Autodesk Inventor part; units mm, degrees
ref_plane "Work Plane7" through (3.7071, 39.9, 0.5) normal (0, 1, 0) x (1, 0, 0)
ref_plane "YZ Plane" through (0, 0, 0) normal (1, 0, 0) x (0, 1, 0)
ref_plane "XZ Plane" through (0, 0, 0) normal (0, 1, 0) x (-1, 0, 0)
ref_plane "Work Plane7" through (3.7071, 39.9, 0.5) normal (0, 1, 0) x (1, 0, 0)
sketch "Sketch4" plane through (3.7071, 39.9, 0.5) normal (0, 1, 0) x (1, 0, 0)
  circle A0 centre (6.2928, -9.3) radius 2.9
  circle A1 centre (6.2928, -9.3) radius 2.65
  line L0 (6.2928, -9.3) -> (6.2928, -8.1563)
  circle A2 centre (6.2928, -9.3) radius 1.5
  line L1 (5.9607, -6.6709) -> (6.3303, -6.4003)
  line L2 (6.6249, -6.6709) -> (6.3303, -6.4003)
  line L3 (5.3173, -6.8361) -> (5.608, -6.482)
  line L4 (5.9607, -6.6709) -> (5.608, -6.482)
  line L5 (4.7352, -7.1561) -> (4.9287, -6.7409)
  line L6 (5.3173, -6.8361) -> (4.9287, -6.7409)
  line L7 (4.2509, -7.6109) -> (4.3351, -7.1605)
  line L8 (4.7352, -7.1561) -> (4.3351, -7.1605)
  line L9 (3.895, -8.1717) -> (3.8646, -7.7146)
  line L10 (4.2509, -7.6109) -> (3.8646, -7.7146)
  line L11 (3.6897, -8.8035) -> (3.5466, -8.3682)
  line L12 (3.895, -8.1717) -> (3.5466, -8.3682)
  line L13 (3.648, -9.4664) -> (3.4011, -9.0805)
  line L14 (3.6897, -8.8035) -> (3.4011, -9.0805)
  line L15 (3.7725, -10.1189) -> (3.4374, -9.8065)
  line L16 (3.648, -9.4664) -> (3.4374, -9.8065)
  line L17 (4.0553, -10.72) -> (3.653, -10.5007)
  line L18 (3.7725, -10.1189) -> (3.653, -10.5007)
  line L19 (4.4787, -11.2318) -> (4.0346, -11.1195)
  line L20 (4.0553, -10.72) -> (4.0346, -11.1195)
  line L21 (5.0161, -11.6222) -> (4.558, -11.6239)
  line L22 (4.4787, -11.2318) -> (4.558, -11.6239)
  line L23 (5.6338, -11.8668) -> (5.1904, -11.9823)
  line L24 (5.0161, -11.6222) -> (5.1904, -11.9823)
  line L25 (6.2928, -11.95) -> (5.8921, -12.1722)
  line L26 (5.6338, -11.8668) -> (5.8921, -12.1722)
  line L27 (6.9518, -11.8668) -> (6.619, -12.1816)
  line L28 (6.2928, -11.95) -> (6.619, -12.1816)
  line L29 (7.5694, -11.6222) -> (7.3254, -12.01)
  line L30 (6.9518, -11.8668) -> (7.3254, -12.01)
  line L31 (8.1068, -11.2318) -> (7.9668, -11.6681)
  line L32 (7.5694, -11.6222) -> (7.9668, -11.6681)
  line L33 (8.5303, -10.72) -> (8.5032, -11.1773)
  line L34 (8.1068, -11.2318) -> (8.5032, -11.1773)
  line L35 (8.8131, -10.1189) -> (8.9006, -10.5687)
  line L36 (8.5303, -10.72) -> (8.9006, -10.5687)
  line L37 (8.9376, -9.4664) -> (9.1341, -9.8803)
  line L38 (8.8131, -10.1189) -> (9.1341, -9.8803)
  line L39 (8.8959, -8.8035) -> (9.1892, -9.1554)
  line L40 (8.9376, -9.4664) -> (9.1892, -9.1554)
  line L41 (8.6906, -8.1717) -> (9.0622, -8.4397)
  line L42 (8.8959, -8.8035) -> (9.0622, -8.4397)
  line L43 (8.3346, -7.6109) -> (8.7613, -7.778)
  line L44 (8.6906, -8.1717) -> (8.7613, -7.778)
  line L45 (7.8504, -7.1561) -> (8.3052, -7.2119)
  line L46 (8.3346, -7.6109) -> (8.3052, -7.2119)
  line L47 (7.2683, -6.8361) -> (7.7227, -6.777)
  line L48 (7.8504, -7.1561) -> (7.7227, -6.777)
  line L49 (6.6249, -6.6709) -> (7.0503, -6.5007)
  line L50 (7.2683, -6.8361) -> (7.0503, -6.5007)
  line L51 (-48.7072, 67.5) -> (-9.1072, 67.5)
  line L52 (-9.1072, 67.5) -> (-9.1072, 47.9)
  line L53 (-9.1072, 47.9) -> (-48.7072, 47.9)
  line L54 (-48.7072, 47.9) -> (-48.7072, 67.5)
  line L55 (-9.6072, 67.8) -> (-48.2072, 67.8)
  line L56 (-49.0072, 67) -> (-49.0072, 48.4)
  line L57 (-48.2072, 47.6) -> (-9.6072, 47.6)
  line L58 (-8.8072, 48.4) -> (-8.8072, 67)
  arc A3 (-48.2072, 67.8) -> (-49.0072, 67) centre (-48.2072, 67) ccw
  arc A4 (-49.0072, 48.4) -> (-48.2072, 47.6) centre (-48.2072, 48.4) ccw
  arc A5 (-8.8072, 67) -> (-9.6072, 67.8) centre (-9.6072, 67) ccw
  arc A6 (-9.6072, 47.6) -> (-8.8072, 48.4) centre (-9.6072, 48.4) ccw
  circle A7 centre (-38.7072, 57.7) radius 2.8043
  line L59 (-28.9072, 67.5) -> (-28.9072, 60.5718)
  arc A8 (-51.4012, 75.2248) -> (-53.5593, 41.3351) centre (-51.641, 58.2265) ccw
  arc A9 (14.1928, -9.3) -> (-1.6072, -9.3) centre (6.2928, -9.3) ccw
  line L60 (-53.5593, 41.3351) -> (-46.7288, 40.1839) construction
  line L61 (-46.7288, 40.1839) -> (-26.4146, 41.3143) construction
  line L62 (-26.4146, 41.3143) -> (-16.8338, 33.5272) construction
  line L63 (-16.8338, 33.5272) -> (-7.2254, 12.1154) construction
  line L64 (-7.2254, 12.1154) -> (-2.9491, -1.4) construction
  line L65 (-2.9491, -1.4) -> (-1.6072, -5.4747) construction
  line L66 (-1.6072, -5.4747) -> (-1.6072, -9.3) construction
  spline S0 degree 4 poles (-53.5593, 41.3351) (-46.7288, 40.1839) (-26.4146, 41.3143) (-16.8338, 33.5272) (-7.2254, 12.1154) (-2.9491, -1.4) (-1.6072, -5.4747) (-1.6072, -9.3) knots 1 1 1 1 1 2 3 4 5 5 5 5 5
  line L67 (61.2928, 67.5) -> (21.6928, 67.5)
  line L68 (21.6928, 67.5) -> (21.6928, 47.9)
  line L69 (21.6928, 47.9) -> (61.2928, 47.9)
  line L70 (61.2928, 47.9) -> (61.2928, 67.5)
  line L71 (22.1928, 67.8) -> (60.7928, 67.8)
  line L72 (61.5928, 67) -> (61.5928, 48.4)
  line L73 (60.7928, 47.6) -> (22.1928, 47.6)
  line L74 (21.3928, 48.4) -> (21.3928, 67)
  arc A10 (61.5928, 67) -> (60.7928, 67.8) centre (60.7928, 67) ccw
  arc A11 (60.7928, 47.6) -> (61.5928, 48.4) centre (60.7928, 48.4) ccw
  arc A12 (22.1928, 67.8) -> (21.3928, 67) centre (22.1928, 67) ccw
  arc A13 (21.3928, 48.4) -> (22.1928, 47.6) centre (22.1928, 48.4) ccw
  circle A14 centre (51.2928, 57.7) radius 2.8043
  line L75 (41.4928, 67.5) -> (41.4928, 60.5718)
  arc A15 (66.1449, 41.3351) -> (63.9868, 75.2248) centre (64.2266, 58.2265) ccw
  line L76 (66.1449, 41.3351) -> (59.3144, 40.1839) construction
  line L77 (59.3144, 40.1839) -> (39.0002, 41.3143) construction
  line L78 (39.0002, 41.3143) -> (29.4194, 33.5272) construction
  line L79 (29.4194, 33.5272) -> (19.811, 12.1154) construction
  line L80 (19.811, 12.1154) -> (15.5347, -1.4) construction
  line L81 (15.5347, -1.4) -> (14.1928, -5.4747) construction
  line L82 (14.1928, -5.4747) -> (14.1928, -9.3) construction
  spline S1 degree 4 poles (66.1449, 41.3351) (59.3144, 40.1839) (39.0002, 41.3143) (29.4194, 33.5272) (19.811, 12.1154) (15.5347, -1.4) (14.1928, -5.4747) (14.1928, -9.3) knots 1 1 1 1 1 2 3 4 5 5 5 5 5
  arc A16 (-1.6072, -9.3) -> (14.1928, -9.3) centre (6.2928, -9.3) ccw
  circle A17 centre (-53.6572, 62.7) radius 1.5
  line L83 (-49.0072, 57.7) -> (-54.6618, 57.7)
  circle A18 centre (-53.6572, 52.7) radius 1.5
  circle A19 centre (66.2428, 62.7) radius 1.5
  circle A20 centre (66.2428, 52.7) radius 1.5
  circle A21 centre (6.2928, -9.3) radius 4.95
  line L84 (-4.1572, 57.7) -> (-3.4323, 57.7)
  circle A22 centre (-4.1572, 57.7) radius 1.5
  circle A23 centre (16.7428, 57.7) radius 1.5
  line L85 (-51.4012, 75.2248) -> (63.9868, 75.2248)
  circle A24 centre (6.2928, -9.3) radius 9.5
  line L86 (-3.2072, -9.3) -> (-3.2072, -6.2163) construction
  line L87 (-3.2072, -6.2163) -> (-3.7947, -2.1829) construction
  line L88 (-3.7947, -2.1829) -> (-5.6572, 5.3052) construction
  line L89 (-5.6572, 5.3052) -> (-8.4358, 13.8026) construction
  spline S2 degree 4 poles (-3.2072, -9.3) (-3.2072, -6.2163) (-3.7947, -2.1829) (-5.6572, 5.3052) (-8.4358, 13.8026) knots 1 1 1 1 1 2 2 2 2 2
  line L90 (15.7928, -9.3) -> (15.7928, -6.2163) construction
  line L91 (15.7928, -6.2163) -> (16.3803, -2.1829) construction
  line L92 (16.3803, -2.1829) -> (18.2428, 5.3052) construction
  line L93 (18.2428, 5.3052) -> (21.0213, 13.8026) construction
  spline S3 degree 4 poles (15.7928, -9.3) (15.7928, -6.2163) (16.3803, -2.1829) (18.2428, 5.3052) (21.0213, 13.8026) knots 1 1 1 1 1 2 2 2 2 2
  line L94 (6.2928, 52.7) -> (6.2928, 2.4423)
  line L95 (6.2928, 33.5913) -> (-0.4039, 33.5913)
  line L96 (-2.3125, 30.9937) -> (6.2928, 3.511)
  arc A25 (-0.4039, 33.5913) -> (-2.3125, 30.9937) centre (-0.4039, 31.5913) ccw
  line L97 (6.2928, 33.5913) -> (12.9895, 33.5913)
  line L98 (14.8981, 30.9937) -> (6.2928, 3.511)
  arc A26 (14.8981, 30.9937) -> (12.9895, 33.5913) centre (12.9895, 31.5913) ccw
  arc A27 (4.7409, 8.4673) -> (7.8447, 8.4673) centre (6.2928, 8.7018) ccw
  point P0 (6.2928, -6.65)
  point P1 (-28.9072, 64.0359)
  point P2 (41.4928, 64.0359)
  point P3 (8.8959, -8.8035)
  point P4 (8.8131, -10.1189)
  point P5 (8.1068, -11.2318)
  point P6 (7.5694, -11.6222)
  point P7 (6.6249, -6.6709)
  point P8 (8.9006, -10.5687)
  point P9 (3.4374, -9.8065)
  point P10 (8.9006, -10.5687)
  point P11 (3.4374, -9.8065)
  point P12 (3.653, -10.5007)
  point P13 (7.9668, -11.6681)
  point P14 (3.653, -10.5007)
  point P15 (7.3254, -12.01)
  point P16 (7.9668, -11.6681)
  point P17 (6.619, -12.1816)
  point P18 (7.3254, -12.01)
  point P19 (6.619, -12.1816)
  point P20 (6.2928, -17.2)
  point P21 (21.0213, 13.8026)
  point P22 (7.7013, 8.0093)
  point P23 (4.8843, 8.0093)
  dimension "d26" = 5.8
  dimension "d105" = 19
  dimension "d31" = 0.25
  dimension "d32" = 3
  dimension "d36" = 360
  dimension "d68" = 45
  dimension "d69" = 67
  dimension "d70" = 39.6
  dimension "d71" = 19.6
  dimension "d72" = 10
  dimension "d73" = 9.8
  dimension "d74" = 0.3
  dimension "d75" = 0.8
  dimension "d78" = 5
  dimension "d91" = 24.75
  dimension "d92" = 3
  dimension "d93" = 5
  dimension "d99" = 9.9
  dimension "d102" = 3
  dimension "d104" = 17
  dimension "d106" = 2
extrude "Extrusion9" add sketch "Sketch4" along normal blind 3 contours L85 A15 S1 A24 S0 A8 | S0 A24 S2 | A24 S1 A9 S0 | S0 A16 S1 A24 | S3 A24 S1 | A9 A16 | A27 L98 L94 | L94 L96 A27 | A27 L96 | L98 A27
properties part number "Shoulder_bottom" material "Thermoplastic Resin"
Part model, mm, in its own coordinate system. A direction names the side the tool comes from. Give positions to 0.01 mm unless a question says otherwise; leave off trailing zeros. Order: outer loops, then holes, each group sorted by start corner. A loop starts at its lowest first (then second) coordinate and runs counter-clockwise, first axis right, second up. Notation, with made-up numbers: (-16.75, 19.25) -> (-4.75, 19.25) arc R6 cw to (-4.75, 27.25) -> close; hole circle Ø2 at (-17, 79). An arc over 180 degrees is marked (long way). Use one line per item in the form item = value.
(1) Tool access for faces 1 (the face through (45, 41, -67.3)), 2 (the face through (10.209, 41.379, 19.298)): list every direction of +Z, -Z, +X, -X, +Y, -Y with a clear straight run to the whole face (end or side of a thin tool).
Solution:
face_1 = +Y, -Y
face_2 = +Z, +Y, -Y
(2) Flat gauge pins, fed straight in: P1, Ø5, axis at x = 29, z = -65, coming from the -Y side; P2, Ø1.5, axis at y = 42, z = -56, coming from the +X side; P3, Ø1.5, axis at x = 36.5, y = 41.5, coming from the +Z side; P4, Ø0.9, axis at x = 7.5, y = 42, coming from the +Z side. Where does each tip first touch, or does it go through?
Solution:
P1 = 39.9
P2 = 84.91
P3 = -32.9
P4 = 19.08
(3) Pull direction Z, two halves, no side cores. Call faces 3 (the face through (-64.92, 41.38, -58.45)), 4 (the face through (9, 41, -74.725)), 5 (the face through (-5.1, 41, -57)), 6 (the face through (45, 41, -47.1)): +Z half, -Z half, draft (parallel to the pull), parting line (faces both ways), or undercut.
Solution:
face_3 = parting line
face_4 = -Z half
face_5 = undercut
face_6 = undercut
(4) Drill centre lines: line 1 (X direction, y = 41.75, z = -57.5); line 2 (X direction, y = 41.9, z = -62.2); line 3 (X direction, y = 41.7, z = 9.8). Where is each one in solid material? Low to high. Write a range as from..to.
Solution:
line_1 = -64.93..-45.3, -5.1..-1.92, 1.02..18.98, 21.92..25.1, 65.3..84.93
line_2 = -64.33..-51.45, -48.45..-45.3, -5.1..25.1, 65.3..68.45, 71.45..84.33
line_3 = 0.5..5.05, 14.95..19.5
(5) Saw through at C-C (z = -52.2). Write the cut outline in (x, y).
Solution:
outline = (-64.01, 39.9) -> (-51.45, 39.9) -> (-51.45, 42.9) -> (-64.01, 42.9) -> close; (-48.45, 39.9) -> (-45.3, 39.9) -> (-45.3, 42.9) -> (-48.45, 42.9) -> close; (-5.1, 39.9) -> (25.1, 39.9) -> (25.1, 42.9) -> (-5.1, 42.9) -> close; (65.3, 39.9) -> (68.45, 39.9) -> (68.45, 42.9) -> (65.3, 42.9) -> close; (71.45, 39.9) -> (84.01, 39.9) -> (84.01, 42.9) -> (71.45, 42.9) -> close
(6) Saw through at B-B (y = 41.6). Count the separate pieces of the cut face and the enclosed holes in it, then the cut area to 3 significant figures.
Solution:
separate_pieces = 1
enclosed_holes = 10
area = 4,810 mm²
(7) Saw through at A-A (z = -62.2). Write the cut outline in (x, y), then the cut area to 3 significant figures.
Solution:
outline = (-64.33, 39.9) -> (-51.45, 39.9) -> (-51.45, 42.9) -> (-64.33, 42.9) -> close; (-48.45, 39.9) -> (-45.3, 39.9) -> (-45.3, 42.9) -> (-48.45, 42.9) -> close; (-5.1, 39.9) -> (25.1, 39.9) -> (25.1, 42.9) -> (-5.1, 42.9) -> close; (65.3, 39.9) -> (68.45, 39.9) -> (68.45, 42.9) -> (65.3, 42.9) -> close; (71.45, 39.9) -> (84.33, 39.9) -> (84.33, 42.9) -> (71.45, 42.9) -> close
area = 187 mm²
